Input: part model. Units: mm. Frame: model coordinates. Face numbers are marked on the shaded views. A direction names the side the tool comes from. Round coordinates to 2 decimals unless told otherwise and drop trailing zeros. Write each loop counter-clockwise with the first axis right and the second up, starting at its lowest first coordinate (ties: lowest second). Pieces come first, ordered by that corner, then holes. Notation, with made-up numbers: M 34,-36.75 L 41,-36.75 A19 cw 41,-22.75 Z; hole C 82.25,23.25 d8. An arc over 180 degrees is marked long. Use one line per item in the form item = value. Start each with the question number.
Autodesk Inventor part; units mm, degrees
ref_plane "ANBAU_XY" through (0, 0, -15.2) normal (0, -1, 0) x (1, 0, 0)
ref_plane "ANBAU_YZ" through (0, 0, -15.2) normal (1, 0, 0) x (0, 0, 1)
ref_plane "ANBAU_ZX" through (0, 0, -15.2) normal (0, 0, 1) x (0, -1, 0)
sketch "Sketch_1" plane through (0, 0, 0) normal (1, 0, 0) x (0, 1, 0)
  line L0 (22, 5.4) -> (-20.8, 5.4)
  arc A0 (-20.8, 5.4) -> (-21, 5.2) centre (-20.8, 5.2) ccw
  line L1 (-21, 5.2) -> (-21, 1.1788)
  arc A1 (-21, 1.1788) -> (-20.9463, 1.0424) centre (-20.8, 1.1788) ccw
  line L2 (-20.9463, 1.0424) -> (-20.419, 0.477)
  arc A2 (-20.419, 0.477) -> (-19.322, 0) centre (-19.322, 1.5) ccw
  line L3 (-19.322, 0) -> (21.2, 0)
  line L4 (21.2, 0) -> (21.2, -3.3)
  line L5 (21.2, -3.3) -> (21.6171, -3.3)
  line L6 (21.6171, -3.3) -> (22.1063, -2.2509)
  arc A3 (22.1063, -2.2509) -> (22.2, -1.8283) centre (21.2, -1.8283) ccw
  line L7 (22.2, -1.8283) -> (22.2, 5.2)
  arc A4 (22.2, 5.2) -> (22, 5.4) centre (22, 5.2) ccw
extrude "Extrusion1" add sketch "Sketch_1" along normal mid plane 8
sketch "Sketch_6" plane through (0, -21.6, 0) normal (0, 1, 0) x (1, 0, 0)
  arc A0 (-1.7301, -0.5774) -> (-2.6364, 0) centre (-2.6364, -1) ccw
  line L0 (-1.7301, -0.5774) -> (-1.2427, -1.6226)
  arc A1 (-1.2427, -1.6226) -> (-0.3364, -2.2) centre (-0.3364, -1.2) ccw
  line L1 (-0.3364, -2.2) -> (0.3364, -2.2)
  arc A2 (0.3364, -2.2) -> (1.2427, -1.6226) centre (0.3364, -1.2) ccw
  line L2 (1.2427, -1.6226) -> (1.7301, -0.5774)
  arc A3 (2.6364, 0) -> (1.7301, -0.5774) centre (2.6364, -1) ccw
  line L3 (2.6364, 0) -> (-2.6364, 0)
extrude "Extrusion2" cut sketch "Sketch_6" along normal blind 42.8
sketch "Sketch_9" plane through (0, 0, 0) normal (0, 0, 1) x (1, 0, 0)
  line L0 (-5, -18.3964) -> (-5, -23.2)
  line L1 (-5, -23.2) -> (5, -23.2)
  line L2 (5, -23.2) -> (5, -18.3964)
  line L3 (5, -18.3964) -> (4, -18.3964)
  arc A0 (3.9732, -18.4964) -> (4, -18.3964) centre (3.8, -18.3964) ccw
  line L4 (3.9732, -18.4964) -> (1.8927, -22.1)
  arc A1 (1.7195, -22.2) -> (1.8927, -22.1) centre (1.7195, -22) ccw
  line L5 (1.7195, -22.2) -> (-1.7195, -22.2)
  arc A2 (-1.8927, -22.1) -> (-1.7195, -22.2) centre (-1.7195, -22) ccw
  line L6 (-1.8927, -22.1) -> (-3.9732, -18.4964)
  arc A3 (-4, -18.3964) -> (-3.9732, -18.4964) centre (-3.8, -18.3964) ccw
  line L7 (-4, -18.3964) -> (-5, -18.3964)
extrude "Extrusion3" cut sketch "Sketch_9" along normal blind 4
sketch "Sketch_11" plane through (0, 0, 5.4) normal (0, 0, 1) x (1, 0, 0)
  line L0 (-2.75, 13.4123) -> (0, 11.8246)
  line L1 (0, 11.8246) -> (2.75, 13.4123)
  line L2 (2.75, 13.4123) -> (2.75, 16.5877)
  line L3 (2.75, 16.5877) -> (0, 18.1754)
  line L4 (0, 18.1754) -> (-2.75, 16.5877)
  line L5 (-2.75, 16.5877) -> (-2.75, 13.4123)
sketch "Sketch_12" plane through (0, 0, 5.4) normal (0, 0, 1) x (1, 0, 0)
  line L0 (-2.75, -16.5877) -> (0, -18.1754)
  line L1 (0, -18.1754) -> (2.75, -16.5877)
  line L2 (2.75, -16.5877) -> (2.75, -13.4123)
  line L3 (2.75, -13.4123) -> (0, -11.8246)
  line L4 (0, -11.8246) -> (-2.75, -13.4123)
  line L5 (-2.75, -13.4123) -> (-2.75, -16.5877)
extrude "Extrusion4" add sketch "Sketch_12" along normal blind 0.4
extrude "Extrusion5" add sketch "Sketch_11" along normal blind 0.4
sketch "Sketch_10" plane through (0, 0, 0) normal (1, 0, 0) x (0, 1, 0)
  line L0 (15, 0) -> (15, 5.8)
  line L1 (15, 5.8) -> (16.5, 5.8)
  line L2 (16.5, 5.8) -> (16.2295, 5.5295)
  line L3 (16.2295, 5.5295) -> (16.2295, 4.2705)
  line L4 (16.2295, 4.2705) -> (16.5, 4)
  line L5 (16.5, 4) -> (16.75, 4)
  line L6 (16.75, 4) -> (16.75, 0)
  line L7 (16.75, 0) -> (15, 0)
  line L8 (15, 0) -> (15, 5.8)
revolve "Revolution1" cut sketch "Sketch_10" angle 360 about axis through (0, 15, 0) along (0, 0, -1)
thread "Thread1"
sketch "Sketch_13" plane through (0, 0, 0) normal (1, 0, 0) x (0, 1, 0)
  line L0 (-15, 0) -> (-15, 5.8)
  line L1 (-15, 5.8) -> (-13.5, 5.8)
  line L2 (-13.5, 5.8) -> (-13.7705, 5.5295)
  line L3 (-13.7705, 5.5295) -> (-13.7705, 4.2705)
  line L4 (-13.7705, 4.2705) -> (-13.5, 4)
  line L5 (-13.5, 4) -> (-13.25, 4)
  line L6 (-13.25, 4) -> (-13.25, 0)
  line L7 (-13.25, 0) -> (-15, 0)
  line L8 (-15, 0) -> (-15, 5.8)
revolve "Revolution2" cut sketch "Sketch_13" angle 360 about axis through (0, -15, 0) along (0, 0, -1)
thread "Thread2"
ref_plane "ANBAU_XY" through (0, 0, -15.2) normal (0, -1, 0) x (1, 0, 0)
ref_plane "ANBAU_YZ" through (0, 0, -15.2) normal (1, 0, 0) x (0, 0, 1)
ref_plane "ANBAU_ZX" through (0, 0, -15.2) normal (0, 0, 1) x (0, -1, 0)
ref_plane "ANBAU_2_XY" through (0, 0, -15.2) normal (1, 0, 0) x (0, 0, -1)
ref_plane "ANBAU_2_YZ" through (0, 0, -15.2) normal (0, 0, -1) x (0, 1, 0)
ref_plane "ANBAU_2_ZX" through (0, 0, -15.2) normal (0, 1, 0) x (1, 0, 0)
ref_plane "IP1_XY" through (0, 0, 5.4) normal (0, 0, -1) x (1, 0, 0)
ref_plane "IP1_YZ" through (0, 0, 5.4) normal (1, 0, 0) x (0, -1, 0)
ref_plane "IP1_ZX" through (0, 0, 5.4) normal (0, -1, 0) x (0, 0, -1)
ref_plane "IP_ANBAU_XY" through (0, 0, 0) normal (0, 0, -1) x (1, 0, 0)
ref_plane "IP_ANBAU_YZ" through (0, 0, 0) normal (1, 0, 0) x (0, -1, 0)
ref_plane "IP_ANBAU_ZX" through (0, 0, 0) normal (0, -1, 0) x (0, 0, -1)
ref_plane "IP_ANBAU_2_XY" through (0, 0, -15.2) normal (1, 0, 0) x (0, 0, -1)
ref_plane "IP_ANBAU_2_YZ" through (0, 0, -15.2) normal (0, 0, -1) x (0, 1, 0)
ref_plane "IP_ANBAU_2_ZX" through (0, 0, -15.2) normal (0, 1, 0) x (1, 0, 0)
properties part number "8116179 MS4-MV-B---(0_high_m)"
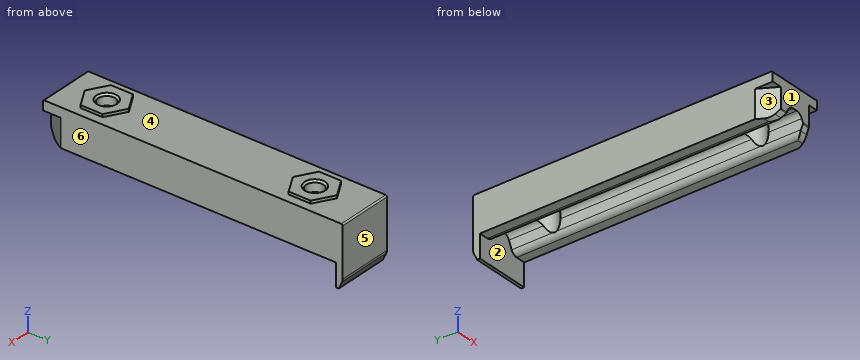
Item 1: Reachability of the marked faces 1, 2 and 3 from +Z, -Z, +X, -X, +Y, -Y: full face, straight path, thin tool, end or side. Return the list, or none.
Item 2: Ray query, line 1 (X direction, y = -15, z = 2); line 2 (Z direction, x = -2.5, y = -0.5); line 3 (X direction, y = 15, z = 5.15). Return the intervals inside material, ascending. Write a range as from..to.
Item 3: Cut plane B-B (y = -7). Output: boundary loops of the cut face in (x, z), plus the area to 3 significant figures.
Item 4: Draft query along Y for the marked faces 4, 5 and 6. Return one class per face: +Y half, -Y half, draft (parallel to the pull), parting line (faces both ways), or undercut.
Item 5: First-contact query: pin 1 (3 mm diameter, centred on x = -1.5, z = 0, fed in from -Y); pin 2 (1 mm diameter, centred on x = -1, z = 0.5, fed in from -Y); pin 3 (4.5 mm diameter, centred on x = 0, y = 15, fed in from -Z); pin 4 (4 mm diameter, centred on x = 0, y = -15, fed in from -Z). Flat tips, straight axial feed; report the tip coordinate or a pass-through.
Item 6: Cut plane A-A (z = 3.5). Output: boundary loops of the cut face in (x, y).
Final values:
q1.face_1 = +Z, -Z, +X, -X, -Y
q1.face_2 = -Z, -Y
q1.face_3 = -Z, -X, -Y
q2.line_1 = -4..-1.75, 1.75..4
q2.line_2 = 0.01..5.4
q2.line_3 = -4..-1.23, 1.23..4
q3.outline = M -4,0 L -2.64,0 A1 ccw -1.73,0.58 L -1.24,1.62 A1 cw -0.34,2.2 L 0.34,2.2 A1 cw 1.24,1.62 L 1.73,0.58 A1 ccw 2.64,0 L 4,0 L 4,5.4 L -4,5.4 Z
q3.area = 36.7 mm^2
q4.face_4 = undercut
q4.face_5 = +Y half
q4.face_6 = draft
q5.pin_1 = -21
q5.pin_2 = 21.2
q5.pin_3 = 0.08
q5.pin_4 = 0.23
q6.outline = M -4,-18.4 A0.2 ccw -3.97,-18.5 L -2.53,-21 L 2.53,-21 L 3.97,-18.5 A0.2 ccw 4,-18.4 L 4,22.2 L -4,22.2 Z; hole C 0,-15 d3.5; hole C 0,15 d3.5
